Check sheet for the modelled part. Datum: model origin and axes. Units: mm. Coordinates: 2 decimals unless noted, no trailing zeros. Write each loop counter-clockwise with the first axis right and the second up, starting at its lowest first coordinate (ties: lowest second). Pieces come first, ordered by that corner, then holes. Notation, with made-up numbers: M -31,27 L 22,27 A19 ccw 22,41 Z; hole C 77.5,2.5 d4. An arc over 180 degrees is marked long. Answer as CSV lines item,"result". Start each with the question number.
1) Section check A-A (y = 0). Record the cut outline in (x, z), and give its area (3 significant figures).
2) Section check B-B (z = -14). Record the cut outline in (x, y).
3) Material ranges on L1, parallel to Z at x = 79, y = 0; L2, parallel to Z at x = 90.5, y = 19; L3, parallel to Y at x = 138.5, z = 33, recorded low to high. Write a range as [from, to].
4) Draft check along Y on faces 1 (the cylindrical face through (74.131, 42.402, 13.353)), 2 (the flat face through (74, -68.381, -1)), 3 (the flat face through (150.368, -47, 0)). Enter one of: +Y half, -Y half, draft (parallel to the pull), parting line (faces both ways), or undercut.
5) Section check C-C (x = 39). Record the cut outline in (y, z).
from build123d import *

# Parameters (mm, degrees)
F0_W     = 135.365754
F0_H     = 108.153057
F0_R     = 44.4552
F1_DEPTH = 150.368


with BuildPart() as f1:
    # F0 (on Right) → F1 (new body)
    with BuildSketch(Plane.YZ):
        with Locations((-0.697762, -0.581467)):
            Rectangle(F0_W, F0_H)
        Circle(F0_R, mode=Mode.SUBTRACT)
    extrude(amount=F1_DEPTH)


solid = f1.part
Results found:
1,outline,"M 0,-54.66 L 150.37,-54.66 L 150.37,-44.46 L 0,-44.46 Z; M 0,44.46 L 150.37,44.46 L 150.37,53.5 L 0,53.5 Z"
1,area,"2,890 mm2"
2,outline,"M 0,-68.38 L 150.37,-68.38 L 150.37,-42.19 L 0,-42.19 Z; M 0,42.19 L 150.37,42.19 L 150.37,66.99 L 0,66.99 Z"
3,L1,"z = [-54.66, -44.46], [44.46, 53.5]"
3,L2,"z = [-54.66, -40.19], [40.19, 53.5]"
3,L3,"y = [-68.38, -29.79], [29.79, 66.99]"
4,face 1,"undercut"
4,face 2,"-Y half"
4,face 3,"draft"
5,outline,"M -68.38,-54.66 L 66.99,-54.66 L 66.99,53.5 L -68.38,53.5 Z; hole C 0,0 d88.91"
